Could you check a few things on this model? Use its own coordinates, in mm. A direction names the side the tool comes from. Round coordinates to 2 decimals unless told otherwise and drop trailing zeros. Loops run counter-clockwise (first coordinate to the right, second up) from the corner with the lowest first, then second, coordinate; pieces in that order, holes last. Notation, with made-up numbers: (-31, -5.5) -> (-23, -5.5) arc R27 ccw to (-23, 33.5) -> close; hole circle Ø2 at (83.5, -6.75). An arc over 180 degrees is marked (long way). Put each result on its own line as item: value. Start each with the question number.
1. Which directions (+Z, -Z, +X, -X, +Y, -Y) give clear straight access to the entire face, cutting with the end or side of a thin tool? Please do faces 1 (the cylindrical face through (14.459, -15.206, 11.493)), 2 (the cylindrical face through (-29.026, -39.229, 5.916)).
2. Imagine slicing it at A-A, the plane y = -68. Please give me the cut outline in (x, z).
3. Imagine slicing it at C-C, the plane x = 0. Please give me the cut outline in (y, z), and give its area (3 significant figures).
4. If we mould it in two halves opening along Y, with no side actions, what happens to faces 3 (the flat face through (-27.036, -14.423, 5.916)), 4 (the flat face through (2.45, -80.83, 5.92)), 5 (the cylindrical face through (12.031, -21.875, 5.423))? For each: pulls with the +Y half, pulls with the -Y half, needs draft (parallel to the pull), parting line crosses it, or undercut.
5. Imagine slicing it at B-B, the plane z = 4.75. Please give me the cut outline in (x, y), and give its area (3 significant figures).
6. I'm going to push flat-ended pins straight in: P1, Ø6, axis at x = -9, y = 6, coming from the +Z side; P2, Ø2, axis at x = 15, z = 1.5, coming from the +Y side; P3, Ø2, axis at x = -8.5, z = 2, coming from the -Y side; P4, Ø7, axis at x = 12.38, y = -19.2, coming from the +Z side. Where does each tip first touch, or does it pass through?
7. Imagine slicing it at D-D, the plane y = -2. Please give me the cut outline in (x, z).
8. I need wall thicknesses on line 1 (Y direction, x = 0, z = 2.75); line 2 (Y direction, x = 3, z = 5.5); line 3 (X direction, y = -9.5, z = 3.5). Which ranges of each line are inside material? Lowest first, please. Write a range as [from, to].
Autodesk Fusion 360 part; units mm, degrees
sketch "Sketch1" plane through (0, 0, 0) normal (0, 0, 1) x (1, 0, 0)
  circle A0 centre (0, 0) radius 14.05
  circle A1 centre (0, 0) radius 18.05
  line L0 (0, 0) -> (0, -50.8) construction
  line L1 (14.7041, -13.2728) -> (-37.5272, -36.0959)
  line L2 (-37.5272, -36.0959) -> (-14.7041, -88.3272)
  line L3 (-14.7041, -88.3272) -> (37.5272, -65.5041)
  line L4 (37.5272, -65.5041) -> (14.7041, -13.2728)
  line L5 (-37.5272, -36.0959) -> (37.5272, -65.5041) construction
  line L6 (14.7041, -13.2728) -> (-14.7041, -88.3272) construction
  circle A2 centre (0, -50.8) radius 25 construction
  line L7 (25, -36.8353) -> (25, -70.978)
  circle A3 centre (0, -50.8) radius 20
  circle A4 centre (12.3824, -19.1982) radius 2.7
  circle A5 centre (-31.6018, -38.4176) radius 2.7
  circle A6 centre (-12.3824, -82.4018) radius 2.7
  circle A7 centre (31.6018, -63.1824) radius 2.7
  line L8 (25, -36.8353) -> (17.7622, 3.2103)
  line L9 (-37.5272, -36.0959) -> (-16.2465, 7.8647)
  circle A8 centre (0, 0) radius 25 construction
  circle A9 centre (12.3824, -19.1982) radius 4.5
  line L10 (25, -60.5957) -> (20.0915, -73.1228)
  point P0 (0, -50.8)
  dimension "d1" = 28.1
  dimension "d2" = 4
  dimension "d3" = 50.8
  dimension "d4" = 57
  dimension "d5" = 57
  dimension "d6" = 57
  dimension "d7" = 50
  dimension "d8" = 40
  dimension "d9" = 5.4
  dimension "d10" = 4.5
  dimension "d11" = 5.4
  dimension "d12" = 5.4
  dimension "d13" = 5.4
  dimension "d14" = 4.5
  dimension "d15" = 4.5
  dimension "d16" = 4.5
  dimension "d19" = 50
extrude "Extrude1" add sketch "Sketch1" along normal blind 12 contours A1 | A1 L1 L4 L8 | A1 L1 L9 | L1 L2 L3 L4 L7 A9 L10 | L1 L4 A9 | A9 | L3 L7 L10
extrude "Extrude2" cut sketch "Sketch1" along normal blind 1 from surface at 11 contours A9
extrude "Extrude3" cut sketch "Sketch1" along normal blind 12 contours L3 L7 L10
Entries:
1. face 1: +Z
1. face 2: +Z, -Z
2. outline: (-23.59, 0) -> (-10.21, 0) -> (-10.21, 12) -> (-23.59, 12) -> close; (10.21, 0) -> (22.1, 0) -> (22.1, 12) -> (10.21, 12) -> close
3. outline: (-81.9, 0) -> (-70.8, 0) -> (-70.8, 12) -> (-81.9, 12) -> close; (-30.8, 0) -> (-14.05, 0) -> (-14.05, 12) -> (-30.8, 12) -> close; (14.05, 0) -> (18.05, 0) -> (18.05, 12) -> (14.05, 12) -> close
3. area: 382 mm^2
4. face 3: pulls with the +Y half
4. face 4: pulls with the -Y half
4. face 5: undercut
5. outline: (-37.53, -36.1) -> (-14.7, -88.33) -> (20.09, -73.12) -> (25, -60.6) -> (25, -36.84) -> (17.76, 3.21) arc R18.05 ccw to (-16.25, 7.86) -> close; hole circle Ø5.4 at (-31.6, -38.42); hole circle Ø40 at (0, -50.8); hole circle Ø5.4 at (-12.38, -82.4); hole circle Ø28.1 at (0, 0); hole circle Ø5.4 at (12.38, -19.2)
5. area: 2,690 mm^2
6. P1: through
6. P2: y = 11.39
6. P3: y = -86.05
6. P4: z = 11
7. outline: (-21.02, 0) -> (-13.91, 0) -> (-13.91, 12) -> (-21.02, 12) -> close; (13.91, 0) -> (18.7, 0) -> (18.7, 12) -> (13.91, 12) -> close
8. line 1: [-81.9, -70.8], [-30.8, -14.05], [14.05, 18.05]
8. line 2: [-80.59, -70.57], [-31.03, -13.73], [13.73, 17.8]
8. line 3: [-24.65, -10.35], [10.35, 20.06]
